```python
from build123d import *

# Parameters (mm, degrees)
F0_R     = 52
F1_DEPTH = 0.1
F2_R     = 2
F3_DEPTH = 0.101


with BuildPart() as f1:
    # F0 (on Top) → F1 (new body)
    with BuildSketch(Plane.XY):
        Circle(F0_R)
    extrude(amount=F1_DEPTH)

    # F2 (on Top) → F3 (cut, through all)
    with BuildSketch(Plane.XY):
        with Locations((48.5, 0)):
            Circle(F2_R)
        with Locations((0, 48.5)):
            Circle(F2_R)
        with Locations((-48.5, 0)):
            Circle(F2_R)
        with Locations((0, -48.5)):
            Circle(F2_R)
    extrude(amount=F3_DEPTH, mode=Mode.SUBTRACT)


solid = f1.part
```
Check sheet for the modelled part. Datum: model origin and axes. Units: mm. Coordinates: 2 decimals unless noted, no trailing zeros. Write each loop counter-clockwise with the first axis right and the second up, starting at its lowest first coordinate (ties: lowest second). Pieces come first, ordered by that corner, then holes. Notation, with made-up numbers: (87, 47.25) -> (112, 47.25) arc R24 cw to (112, 75.25) -> close; hole circle Ø3 at (-35, -35). An arc over 180 degrees is marked (long way). Use a Markdown table: item, result.
1. Go/stop test with a flat-tipped pin: pin 1 Ø3 at (x, y) = (0, -48.5) entering from +Z. Record where the tip stops, or that it passes through.
Reported:
| item | result |
|---|---|
| pin 1 | passes through |
2. Sectioned sample at C-C (z = 0.05). Enter the section's corners in (x, y).
Reported:
| item | result |
|---|---|
| outline | circle Ø104 at (0, 0); hole circle Ø4 at (-48.5, 0); hole circle Ø4 at (0, -48.5); hole circle Ø4 at (0, 48.5); hole circle Ø4 at (48.5, 0) |
3. Scan lines: line 1 along Y through (x, z) = (42.5, 0.05); line 2 along Y through (x, z) = (26.5, 0.05); line 3 along X through (y, z) = (-22.5, 0.05). Record each from-to range of solid material in increasing order.
Reported:
| item | result |
|---|---|
| line 1 | y = -29.96 to 29.96 |
| line 2 | y = -44.74 to 44.74 |
| line 3 | x = -46.88 to 46.88 |
4. Sectioned sample at B-B (y = -48.5). Enter the section's corners in (x, z) (3 decimals).
Reported:
| item | result |
|---|---|
| outline | (-18.755, 0) -> (-2, 0) -> (-2, 0.1) -> (-18.755, 0.1) -> close; (2, 0) -> (18.755, 0) -> (18.755, 0.1) -> (2, 0.1) -> close |
5. Sectioned sample at A-A (x = 0). Enter the section's corners in (y, z).
Reported:
| item | result |
|---|---|
| outline | (-52, 0) -> (-50.5, 0) -> (-50.5, 0.1) -> (-52, 0.1) -> close; (-46.5, 0) -> (46.5, 0) -> (46.5, 0.1) -> (-46.5, 0.1) -> close; (50.5, 0) -> (52, 0) -> (52, 0.1) -> (50.5, 0.1) -> close |
